```python
from build123d import *

# Parameters (mm, degrees)
F0_R     = 8.5
F0_R_2   = 4
F1_DEPTH = 1.5
F2_DEPTH = 6
F0_R_3   = 12.5
F0_R_4   = 11.15
F3_DEPTH = 1.5
F4_DEPTH = 12
F5_R     = 12.5
F6_DEPTH = 3


with BuildPart() as f1:
    # F0 (on Top) → F1 (new body)
    with BuildSketch(Plane.XY):
        Circle(F0_R)
        Circle(F0_R_2, mode=Mode.SUBTRACT)
    extrude(amount=F1_DEPTH)

    # F0 (on Top) → F2 (join)
    with BuildSketch(Plane.XY):
        Circle(F0_R_2)
    extrude(amount=F2_DEPTH)

    # F0 (on Top) → F3 (join)
    with BuildSketch(Plane.XY):
        Circle(F0_R_3)
        Circle(F0_R_4, mode=Mode.SUBTRACT)
        Circle(F0_R_4)
        Circle(F0_R, mode=Mode.SUBTRACT)
    extrude(amount=F3_DEPTH)

    # F0 (on Top) → F4 (join)
    with BuildSketch(Plane.XY):
        Circle(F0_R_3)
        Circle(F0_R_4, mode=Mode.SUBTRACT)
    extrude(amount=-F4_DEPTH)

    # F5 (on face) → F6 (join)
    with BuildSketch(Plane(origin=(0, 0, -12), x_dir=(1, 0, 0), z_dir=(0, 0, -1))):
        Circle(F5_R)
    extrude(amount=F6_DEPTH)


solid = f1.part
```
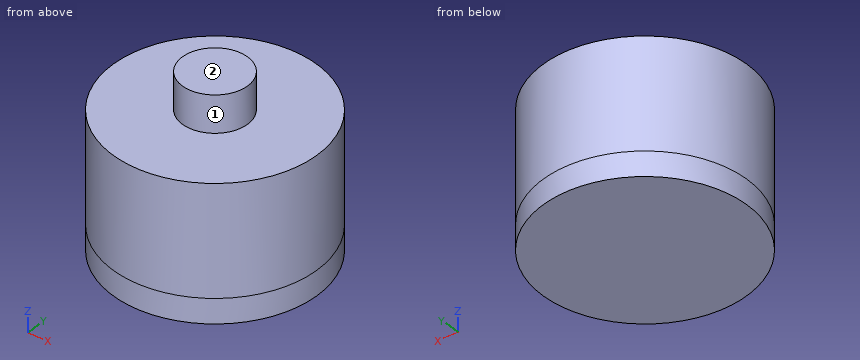
Read the model definition and answer for the solid it produces. Units are mm, in the model's axes. Face numbers are marked on the shaded views. A direction names the side the tool comes from. Give positions to 0.01 mm unless a question says otherwise; leave off trailing zeros. Write each loop counter-clockwise with the first axis right and the second up, starting at its lowest first coordinate (ties: lowest second). Pieces come first, ordered by that corner, then holes. Notation, with made-up numbers: M 56.5,54 L 99.5,54 A7 ccw 99.5,65 Z; hole C 66,-32 d6. An arc over 180 degrees is marked long. Put each result on its own line as item: value. Start each with the question number.
1. The part is cut by section A-A, the plane x = 0. Give the vertices of the cut face in (y, z).
2. Each of these flat-tipped pins is pushed along its axis until it touches: pin 1 Ø2 at (y, z) = (4, -8) entering from -X; pin 2 Ø2 at (x, z) = (-4.5, -12) entering from -Y; pin 3 Ø5 at (y, z) = (-6.5, -3) entering from +X; pin 4 Ø10 at (y, z) = (-1, -5.5) entering from +X. Where does it stop, or does it pass through?
3. The part is cut by section C-C, the plane z = -1. Give the vertices of the cut face in (x, y).
4. The part is cut by section D-D, the plane z = -13. Give the vertices of the cut face in (x, y).
5. Which of the six approach directions +Z, -Z, +X, -X, +Y, -Y give full straight-line access (tool end or side, diameter ignored) to the marked faces 1 and 2?
6. Consider line 1 along Z through (x, y) = (6.5, 7); line 2 along Y through (x, z) = (0, -3.25); line 3 along Z through (x, y) = (-1.75, 1.75). Determine where each line is inside the solid, lowest interval first.
Final values:
1. outline: M -12.5,-15 L 12.5,-15 L 12.5,1.5 L 4,1.5 L 4,6 L -4,6 L -4,1.5 L -12.5,1.5 Z; hole M -11.15,-12 L 11.15,-12 L 11.15,0 L -11.15,0 Z
2. pin 1: stops at x = -12.13
2. pin 2: stops at y = -12
2. pin 3: stops at x = 11.84
2. pin 4: stops at x = 12.5
3. outline: C 0,0 d25; hole C 0,0 d22.3
4. outline: C 0,0 d25
5. face 1: +Z
5. face 2: +Z, +X, -X, +Y, -Y
6. line 1: z = -15 to -12, 0 to 1.5
6. line 2: y = -12.5 to -11.15, 11.15 to 12.5
6. line 3: z = -15 to -12, 0 to 6
